Can you work these out from the model? Positions are in its coordinate system, mm. A direction names the side the tool comes from. Give positions to 0.01 mm unless a question says otherwise; leave off trailing zeros. Loops run counter-clockwise (first coordinate to the right, second up) from the corner with the lowest first, then second, coordinate; pieces in that order, holes last. Notation, with made-up numbers: M 68.25,8.25 L 115.25,8.25 A17 cw 115.25,23.25 Z; hole C -17.75,57.5 d11. An arc over 180 degrees is marked long. One line per item, written item: value. Start each with the question number.
from build123d import *

# Parameters (mm, degrees)
SKETCH1_W           = 300
SKETCH1_H           = 300
SKETCH1_R           = 2.5
SKETCH1_W_2         = 50
SKETCH1_H_2         = 140
BOSS_EXTRUDE1_DEPTH = 5
CUT_EXTRUDE1_START  = -5
SKETCH2_R           = 2.5
CUT_EXTRUDE1_DEPTH  = 5
FILLET1_R           = 10
FILLET2_R           = 50
SKETCH3_W           = 10
SKETCH3_H           = 20
CUT_EXTRUDE2_DEPTH  = 213.190951739
CUT_EXTRUDE3_REACH  = 214.191
SKETCH4_R           = 1.5


with BuildPart() as part:
    # Sketch1 → Boss-Extrude1 (new body)
    with BuildSketch(Plane.XY):
        Rectangle(SKETCH1_W, SKETCH1_H)
        with Locations((42, 47.5)):
            Circle(SKETCH1_R, mode=Mode.SUBTRACT)
        with Locations((42, 32.5)):
            Circle(SKETCH1_R, mode=Mode.SUBTRACT)
        with Locations((60, 32.5)):
            Circle(SKETCH1_R, mode=Mode.SUBTRACT)
        with Locations((60, 47.5)):
            Circle(SKETCH1_R, mode=Mode.SUBTRACT)
        with Locations((-60, 47.5)):
            Circle(SKETCH1_R, mode=Mode.SUBTRACT)
        with Locations((-60, 32.5)):
            Circle(SKETCH1_R, mode=Mode.SUBTRACT)
        with Locations((-42, 32.5)):
            Circle(SKETCH1_R, mode=Mode.SUBTRACT)
        with Locations((-42, 47.5)):
            Circle(SKETCH1_R, mode=Mode.SUBTRACT)
        with Locations((98, 40)):
            Rectangle(SKETCH1_W_2, SKETCH1_H_2, mode=Mode.SUBTRACT)
        with Locations((-98, 40)):
            Rectangle(SKETCH1_W_2, SKETCH1_H_2, mode=Mode.SUBTRACT)
    extrude(amount=BOSS_EXTRUDE1_DEPTH)

    # Sketch2 → Cut-Extrude1 (cut)
    with BuildSketch(Plane.XY.offset(5).offset(CUT_EXTRUDE1_START)):
        with Locations((-60, 32.5)):
            Circle(SKETCH2_R)
        with Locations((-78.125, -90.6)):
            Circle(SKETCH2_R)
        with Locations((-41.875, -90.6)):
            Circle(SKETCH2_R)
        with Locations((-41.875, -119.4)):
            Circle(SKETCH2_R)
        with Locations((-78.125, -119.4)):
            Circle(SKETCH2_R)
        with Locations((78.125, -119.4)):
            Circle(SKETCH2_R)
        with Locations((41.875, -119.4)):
            Circle(SKETCH2_R)
        with Locations((41.875, -90.6)):
            Circle(SKETCH2_R)
        with Locations((78.125, -90.6)):
            Circle(SKETCH2_R)
    extrude(amount=CUT_EXTRUDE1_DEPTH, mode=Mode.SUBTRACT)

    # Fillet1
    fillet1_edges = [part.edges().sort_by_distance(p)[0] for p in [
        (-123, -30, 2.5),
        (-73, -30, 2.5),
        (-73, 110, 2.5),
        (-123, 110, 2.5),
        (73, -30, 2.5),
        (123, -30, 2.5),
        (123, 110, 2.5),
        (73, 110, 2.5),
    ]]
    fillet(fillet1_edges, radius=FILLET1_R)

    # Fillet2
    fillet2_edges = [part.edges().sort_by_distance(p)[0] for p in [
        (150, -150, 2.5),
        (-150, -150, 2.5),
        (-150, 150, 2.5),
        (150, 150, 2.5),
    ]]
    fillet(fillet2_edges, radius=FILLET2_R)

    # Sketch3 → Cut-Extrude2 (cut, through all)
    with BuildSketch(Plane.XY.offset(5)):
        with Locations((-7, 40)):
            Rectangle(SKETCH3_W, SKETCH3_H)
        with BuildLine():
            ThreePointArc((-12, 50), (-7, 55), (-2, 50))
            Line((-2, 50), (-12, 50))
        make_face()
        with BuildLine():
            Line((-12, 30), (-2, 30))
            ThreePointArc((-2, 30), (-7, 25), (-12, 30))
        make_face()
        with BuildLine():
            ThreePointArc((12, 30), (7, 25), (2, 30))
            Line((2, 30), (2, 50))
            ThreePointArc((2, 50), (7, 55), (12, 50))
            Line((12, 50), (12, 30))
        make_face()
    extrude(amount=-CUT_EXTRUDE2_DEPTH, mode=Mode.SUBTRACT)

    # Sketch4 → Cut-Extrude3 (cut, up to next)
    with BuildSketch(Plane.XY.offset(5), mode=Mode.PRIVATE) as cut_extrude3_sk1:
        with Locations((-70, -140)):
            Circle(SKETCH4_R)
    cut_extrude3_tool1 = extrude(cut_extrude3_sk1.sketch, amount=-CUT_EXTRUDE3_REACH, mode=Mode.PRIVATE) & part.part
    # Sketch4 → Cut-Extrude3 (cut, up to next)
    with BuildSketch(Plane.XY.offset(5), mode=Mode.PRIVATE) as cut_extrude3_sk2:
        with Locations((70, -140)):
            Circle(SKETCH4_R)
    cut_extrude3_tool2 = extrude(cut_extrude3_sk2.sketch, amount=-CUT_EXTRUDE3_REACH, mode=Mode.PRIVATE) & part.part
    # Sketch4 → Cut-Extrude3 (cut, up to next)
    with BuildSketch(Plane.XY.offset(5), mode=Mode.PRIVATE) as cut_extrude3_sk3:
        with Locations((-90, -140)):
            Circle(SKETCH4_R)
    cut_extrude3_tool3 = extrude(cut_extrude3_sk3.sketch, amount=-CUT_EXTRUDE3_REACH, mode=Mode.PRIVATE) & part.part
    # Sketch4 → Cut-Extrude3 (cut, up to next)
    with BuildSketch(Plane.XY.offset(5), mode=Mode.PRIVATE) as cut_extrude3_sk4:
        with Locations((90, -140)):
            Circle(SKETCH4_R)
    cut_extrude3_tool4 = extrude(cut_extrude3_sk4.sketch, amount=-CUT_EXTRUDE3_REACH, mode=Mode.PRIVATE) & part.part
    # Sketch4 → Cut-Extrude3 (cut, up to next)
    with BuildSketch(Plane.XY.offset(5), mode=Mode.PRIVATE) as cut_extrude3_sk5:
        with Locations((90, 140)):
            Circle(SKETCH4_R)
    cut_extrude3_tool5 = extrude(cut_extrude3_sk5.sketch, amount=-CUT_EXTRUDE3_REACH, mode=Mode.PRIVATE) & part.part
    # Sketch4 → Cut-Extrude3 (cut, up to next)
    with BuildSketch(Plane.XY.offset(5), mode=Mode.PRIVATE) as cut_extrude3_sk6:
        with Locations((-90, 140)):
            Circle(SKETCH4_R)
    cut_extrude3_tool6 = extrude(cut_extrude3_sk6.sketch, amount=-CUT_EXTRUDE3_REACH, mode=Mode.PRIVATE) & part.part
    # Sketch4 → Cut-Extrude3 (cut, up to next)
    with BuildSketch(Plane.XY.offset(5), mode=Mode.PRIVATE) as cut_extrude3_sk7:
        with Locations((70, 140)):
            Circle(SKETCH4_R)
    cut_extrude3_tool7 = extrude(cut_extrude3_sk7.sketch, amount=-CUT_EXTRUDE3_REACH, mode=Mode.PRIVATE) & part.part
    # Sketch4 → Cut-Extrude3 (cut, up to next)
    with BuildSketch(Plane.XY.offset(5), mode=Mode.PRIVATE) as cut_extrude3_sk8:
        with Locations((-70, 140)):
            Circle(SKETCH4_R)
    cut_extrude3_tool8 = extrude(cut_extrude3_sk8.sketch, amount=-CUT_EXTRUDE3_REACH, mode=Mode.PRIVATE) & part.part
    add(cut_extrude3_tool1.solids().sort_by_distance((-70, -140, 5))[0], mode=Mode.SUBTRACT)
    add(cut_extrude3_tool2.solids().sort_by_distance((70, -140, 5))[0], mode=Mode.SUBTRACT)
    add(cut_extrude3_tool3.solids().sort_by_distance((-90, -140, 5))[0], mode=Mode.SUBTRACT)
    add(cut_extrude3_tool4.solids().sort_by_distance((90, -140, 5))[0], mode=Mode.SUBTRACT)
    add(cut_extrude3_tool5.solids().sort_by_distance((90, 140, 5))[0], mode=Mode.SUBTRACT)
    add(cut_extrude3_tool6.solids().sort_by_distance((-90, 140, 5))[0], mode=Mode.SUBTRACT)
    add(cut_extrude3_tool7.solids().sort_by_distance((70, 140, 5))[0], mode=Mode.SUBTRACT)
    add(cut_extrude3_tool8.solids().sort_by_distance((-70, 140, 5))[0], mode=Mode.SUBTRACT)


solid = part.part
Q1. If we mould it in two halves opening along Y, with no side actions, what happens to faces 3 (the face through (-119.99, -27.15, 2.54)), 4 (the face through (-135.742, -134.964, 2.535)), 5 (the face through (134.964, 135.742, 2.535))? For each: released by +Y, released by -Y, zero draft, split by the parting line, or undercut.
Q2. I need wall thicknesses on line 1 along Y through (x, z) = (-60, 2.35); line 2 along Y through (x, z) = (90, 1.8); line 3 along Y through (x, z) = (70, 1). Which ranges of each line are inside material? Lowest first, please.
Q3. Which directions (+Z, -Z, +X, -X, +Y, -Y) give clear straight access to the entire face, cutting with the end or side of a thin tool? Please do faces 1 (the face through (-2, 2, 0)), 2 (the face through (120.15, 106.99, 2.54)).
Q4. If we section it at B-B, the plane x = 119.5: Write out the boundary of the cut face in (y, z).
Q5. If we section it at D-D, the plane x = -119: Write out the boundary of the cut face in (y, z).
Q6. If we section it at C-C, the plane z = 1.5: Give the number of separate pieces and of enclosed holes in the cut face, plus the area to 3 significant figures.
Q7. If we section it at A-A, the plane y = 18: Write out the boundary of the cut face in (x, z), plus the area to 3 significant figures.
Response:
1. face 3: undercut
1. face 4: released by -Y
1. face 5: released by +Y
2. line 1: -150 to 30, 35 to 45, 50 to 150
2. line 2: -150 to -141.5, -138.5 to -30, 110 to 138.5, 141.5 to 150
2. line 3: -150 to -141.5, -138.5 to 138.5, 141.5 to 150
3. face 1: -Z, +X, -X, +Y, -Y
3. face 2: +Z, -Z
4. outline: M -146.04,0 L -27.6,0 L -27.6,5 L -146.04,5 Z; M 107.6,0 L 146.04,0 L 146.04,5 L 107.6,5 Z
5. outline: M -146.25,0 L -28,0 L -28,5 L -146.25,5 Z; M 108,0 L 146.25,0 L 146.25,5 L 108,5 Z
6. separate pieces: 1
6. enclosed holes: 28
6. area: 73,100 mm^2
7. outline: M -150,0 L -123,0 L -123,5 L -150,5 Z; M -73,0 L 73,0 L 73,5 L -73,5 Z; M 123,0 L 150,0 L 150,5 L 123,5 Z
7. area: 1,000 mm^2
